Read the model definition and answer for the solid it produces. Units are mm, in the model's axes. Give positions to 0.01 mm unless a question says otherwise; leave off trailing zeros. Order: outer loops, then holes, each group sorted by start corner. A loop starts at its lowest first (then second) coordinate and runs counter-clockwise, first axis right, second up.
```python
from build123d import *

# Parameters (mm, degrees)
SKETCH1_W           = 203.2
SKETCH1_H           = 133.35
BOSS_EXTRUDE1_DEPTH = 3.175
SKETCH3_W           = 35.687
SKETCH3_H           = 3.175
BOSS_EXTRUDE2_DEPTH = 3.175
SKETCH4_W           = 3.175
SKETCH4_H           = 18.542
BOSS_EXTRUDE3_DEPTH = 3.175
SKETCH5_W           = 63.5
SKETCH5_H           = 139.7
SKETCH5_R           = 3.429
BOSS_EXTRUDE4_DEPTH = 3.175
BOSS_EXTRUDE5_DEPTH = 3.175
SKETCH7_W           = 3.683
SKETCH7_H           = 19.558
CUT_EXTRUDE1_DEPTH  = 183.223979624
SKETCH8_W           = 71.12
SKETCH8_H           = 45.72
CUT_EXTRUDE4_DEPTH  = 183.223979624


with BuildPart() as part:
    # Sketch1 → Boss-Extrude1 (new body)
    with BuildSketch(Plane(origin=(0, 0, 0), x_dir=(1, 0, 0), z_dir=(0, 1, 0))):
        Rectangle(SKETCH1_W, SKETCH1_H)
    extrude(amount=BOSS_EXTRUDE1_DEPTH)

    # Sketch3 → Boss-Extrude2 (add)
    with BuildSketch(Plane(origin=(0, 3.175, 0), x_dir=(1, 0, 0), z_dir=(0, 1, 0))):
        with Locations((-61.2775, 68.2625)):
            Rectangle(SKETCH3_W, SKETCH3_H)
        with Locations((0.3175, 68.2625)):
            Rectangle(SKETCH3_W, SKETCH3_H)
        with Locations((61.9125, 68.2625)):
            Rectangle(SKETCH3_W, SKETCH3_H)
        with Locations((61.9125, -68.2625)):
            Rectangle(SKETCH3_W, SKETCH3_H)
        with Locations((0.3175, -68.2625)):
            Rectangle(SKETCH3_W, SKETCH3_H)
        with Locations((-61.2775, -68.2625)):
            Rectangle(SKETCH3_W, SKETCH3_H)
    extrude(amount=-BOSS_EXTRUDE2_DEPTH)

    # Sketch4 → Boss-Extrude3 (add)
    with BuildSketch(Plane(origin=(0, 3.175, 0), x_dir=(1, 0, 0), z_dir=(0, 1, 0))):
        with Locations((-103.1875, 38.1)):
            Rectangle(SKETCH4_W, SKETCH4_H)
        with Locations((-103.1875, 0)):
            Rectangle(SKETCH4_W, SKETCH4_H)
        with Locations((-103.1875, -38.1)):
            Rectangle(SKETCH4_W, SKETCH4_H)
        with Locations((103.1875, -38.1)):
            Rectangle(SKETCH4_W, SKETCH4_H)
        with Locations((103.1875, 0)):
            Rectangle(SKETCH4_W, SKETCH4_H)
        with Locations((103.1875, 38.1)):
            Rectangle(SKETCH4_W, SKETCH4_H)
    extrude(amount=-BOSS_EXTRUDE3_DEPTH)

    # Sketch5 → Boss-Extrude4 (add)
    with BuildSketch(Plane(origin=(0, 3.175, 0), x_dir=(1, 0, 0), z_dir=(0, 1, 0))):
        with Locations((-136.525, 0)):
            Rectangle(SKETCH5_W, SKETCH5_H)
        with Locations(Location((-117.475, 57.15, 0), (0, 0, 270))):
            Circle(SKETCH5_R, mode=Mode.SUBTRACT)
        with Locations(Location((-130.175, 57.15, 0), (0, 0, 270))):
            Circle(SKETCH5_R, mode=Mode.SUBTRACT)
        with Locations(Location((-142.875, 57.15, 0), (0, 0, 270))):
            Circle(SKETCH5_R, mode=Mode.SUBTRACT)
        with Locations(Location((-155.575, 57.15, 0), (0, 0, 270))):
            Circle(SKETCH5_R, mode=Mode.SUBTRACT)
        with Locations(Location((-130.175, 44.45, 0), (0, 0, 270))):
            Circle(SKETCH5_R, mode=Mode.SUBTRACT)
        with Locations(Location((-142.875, 44.45, 0), (0, 0, 270))):
            Circle(SKETCH5_R, mode=Mode.SUBTRACT)
        with Locations(Location((-155.575, 44.45, 0), (0, 0, 270))):
            Circle(SKETCH5_R, mode=Mode.SUBTRACT)
        with Locations(Location((-130.175, 31.75, 0), (0, 0, 270))):
            Circle(SKETCH5_R, mode=Mode.SUBTRACT)
        with Locations(Location((-142.875, 31.75, 0), (0, 0, 270))):
            Circle(SKETCH5_R, mode=Mode.SUBTRACT)
        with Locations(Location((-155.575, 31.75, 0), (0, 0, 270))):
            Circle(SKETCH5_R, mode=Mode.SUBTRACT)
        with Locations(Location((-130.175, 19.05, 0), (0, 0, 270))):
            Circle(SKETCH5_R, mode=Mode.SUBTRACT)
        with Locations(Location((-142.875, 19.05, 0), (0, 0, 270))):
            Circle(SKETCH5_R, mode=Mode.SUBTRACT)
        with Locations(Location((-155.575, 19.05, 0), (0, 0, 270))):
            Circle(SKETCH5_R, mode=Mode.SUBTRACT)
        with Locations(Location((-130.175, 6.35, 0), (0, 0, 270))):
            Circle(SKETCH5_R, mode=Mode.SUBTRACT)
        with Locations(Location((-142.875, 6.35, 0), (0, 0, 270))):
            Circle(SKETCH5_R, mode=Mode.SUBTRACT)
        with Locations(Location((-155.575, 6.35, 0), (0, 0, 270))):
            Circle(SKETCH5_R, mode=Mode.SUBTRACT)
        with Locations(Location((-130.175, -6.35, 0), (0, 0, 270))):
            Circle(SKETCH5_R, mode=Mode.SUBTRACT)
        with Locations(Location((-142.875, -6.35, 0), (0, 0, 270))):
            Circle(SKETCH5_R, mode=Mode.SUBTRACT)
        with Locations(Location((-155.575, -6.35, 0), (0, 0, 270))):
            Circle(SKETCH5_R, mode=Mode.SUBTRACT)
        with Locations(Location((-130.175, -19.05, 0), (0, 0, 270))):
            Circle(SKETCH5_R, mode=Mode.SUBTRACT)
        with Locations(Location((-142.875, -19.05, 0), (0, 0, 270))):
            Circle(SKETCH5_R, mode=Mode.SUBTRACT)
        with Locations(Location((-155.575, -19.05, 0), (0, 0, 270))):
            Circle(SKETCH5_R, mode=Mode.SUBTRACT)
        with Locations(Location((-130.175, -31.75, 0), (0, 0, 270))):
            Circle(SKETCH5_R, mode=Mode.SUBTRACT)
        with Locations(Location((-142.875, -31.75, 0), (0, 0, 270))):
            Circle(SKETCH5_R, mode=Mode.SUBTRACT)
        with Locations(Location((-155.575, -31.75, 0), (0, 0, 270))):
            Circle(SKETCH5_R, mode=Mode.SUBTRACT)
        with Locations(Location((-130.175, -44.45, 0), (0, 0, 270))):
            Circle(SKETCH5_R, mode=Mode.SUBTRACT)
        with Locations(Location((-142.875, -44.45, 0), (0, 0, 270))):
            Circle(SKETCH5_R, mode=Mode.SUBTRACT)
        with Locations(Location((-155.575, -44.45, 0), (0, 0, 270))):
            Circle(SKETCH5_R, mode=Mode.SUBTRACT)
        with Locations(Location((-130.175, -57.15, 0), (0, 0, 270))):
            Circle(SKETCH5_R, mode=Mode.SUBTRACT)
        with Locations(Location((-142.875, -57.15, 0), (0, 0, 270))):
            Circle(SKETCH5_R, mode=Mode.SUBTRACT)
        with Locations(Location((-155.575, -57.15, 0), (0, 0, 270))):
            Circle(SKETCH5_R, mode=Mode.SUBTRACT)
        with Locations(Location((-117.475, 44.45, 0), (0, 0, 270))):
            Circle(SKETCH5_R, mode=Mode.SUBTRACT)
        with Locations(Location((-117.475, 31.75, 0), (0, 0, 270))):
            Circle(SKETCH5_R, mode=Mode.SUBTRACT)
        with Locations(Location((-117.475, 19.05, 0), (0, 0, 270))):
            Circle(SKETCH5_R, mode=Mode.SUBTRACT)
        with Locations(Location((-117.475, 6.35, 0), (0, 0, 270))):
            Circle(SKETCH5_R, mode=Mode.SUBTRACT)
        with Locations(Location((-117.475, -6.35, 0), (0, 0, 270))):
            Circle(SKETCH5_R, mode=Mode.SUBTRACT)
        with Locations(Location((-117.475, -19.05, 0), (0, 0, 270))):
            Circle(SKETCH5_R, mode=Mode.SUBTRACT)
        with Locations(Location((-117.475, -31.75, 0), (0, 0, 270))):
            Circle(SKETCH5_R, mode=Mode.SUBTRACT)
        with Locations(Location((-117.475, -44.45, 0), (0, 0, 270))):
            Circle(SKETCH5_R, mode=Mode.SUBTRACT)
        with Locations(Location((-117.475, -57.15, 0), (0, 0, 270))):
            Circle(SKETCH5_R, mode=Mode.SUBTRACT)
    extrude(amount=-BOSS_EXTRUDE4_DEPTH)

    # Sketch6 → Boss-Extrude5 (add)
    with BuildSketch(Plane(origin=(0, 3.175, 0), x_dir=(1, 0, 0), z_dir=(0, 1, 0))):
        Polygon((-79.121, 66.675), (-79.121, 69.85), (-104.775, 69.85), (-104.775, 58.6105), (-104.775, 47.371), (-101.6, 47.371), (-101.6, 66.675), align=None)
        Polygon((-104.775, -47.371), (-104.775, -58.6105), (-104.775, -69.85), (-79.121, -69.85), (-79.121, -66.675), (-101.6, -66.675), (-101.6, -47.371), align=None)
        Polygon((79.121, -66.675), (79.121, -69.85), (104.775, -69.85), (104.775, -58.6105), (104.775, -47.371), (101.6, -47.371), (101.6, -66.675), align=None)
        Polygon((104.775, 47.371), (104.775, 58.6105), (104.775, 69.85), (79.121, 69.85), (79.121, 66.675), (101.6, 66.675), (101.6, 47.371), align=None)
    extrude(amount=-BOSS_EXTRUDE5_DEPTH)

    # Sketch7 → Cut-Extrude1 (cut, through all)
    with BuildSketch(Plane(origin=(0, 3.175, 0), x_dir=(1, 0, 0), z_dir=(0, 1, 0))):
        with Locations((-103.1875, 19.05)):
            Rectangle(SKETCH7_W, SKETCH7_H)
        with Locations((-103.1875, -19.05)):
            Rectangle(SKETCH7_W, SKETCH7_H)
    extrude(amount=-CUT_EXTRUDE1_DEPTH, mode=Mode.SUBTRACT)

    # Sketch8 → Cut-Extrude4 (cut, through all)
    with BuildSketch(Plane(origin=(0, 0, 0), x_dir=(1, 0, 0), z_dir=(0, 1, 0))):
        with Locations((50.8, 0)):
            Rectangle(SKETCH8_W, SKETCH8_H)
    extrude(amount=CUT_EXTRUDE4_DEPTH, mode=Mode.SUBTRACT)


solid = part.part
```
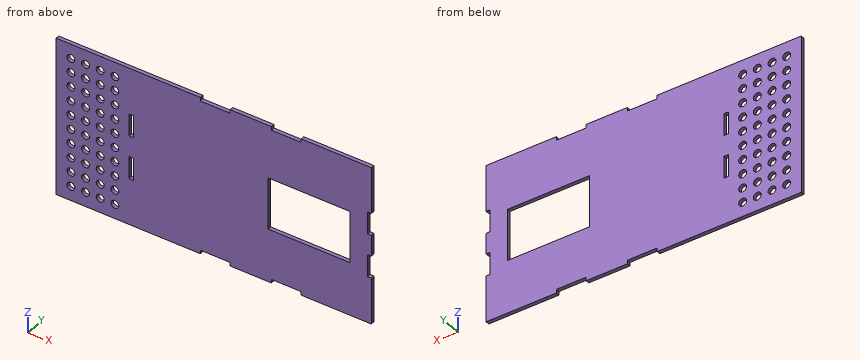
1) The part is cut by section B-B on z = 19.05. Determine the outline of the cut face in (x, y) (3 decimals).
Final values:
outline: (-168.275, 0) - (-159.004, 0) - (-159.004, 3.175) - (-168.275, 3.175) - close; (-152.146, 0) - (-146.304, 0) - (-146.304, 3.175) - (-152.146, 3.175) - close; (-139.446, 0) - (-133.604, 0) - (-133.604, 3.175) - (-139.446, 3.175) - close; (-126.746, 0) - (-120.904, 0) - (-120.904, 3.175) - (-126.746, 3.175) - close; (-114.046, 0) - (-105.029, 0) - (-105.029, 3.175) - (-114.046, 3.175) - close; (-101.346, 0) - (15.24, 0) - (15.24, 3.175) - (-101.346, 3.175) - close; (86.36, 0) - (101.6, 0) - (101.6, 3.175) - (86.36, 3.175) - close
2) The part is cut by section A-A on x = 21.5. Determine the outline of the cut face in (y, z) (3 decimals).
Final values:
outline: (0, -66.675) - (3.175, -66.675) - (3.175, -22.86) - (0, -22.86) - close; (0, 22.86) - (3.175, 22.86) - (3.175, 66.675) - (0, 66.675) - close
3) Consider L1, parallel to X at y = 0.85, z = -6.35 (3 decimals); L2, parallel to X at y = 1.8, z = 44.45 (3 decimals); L3, parallel to X at y = 0.15, z = 12 (3 decimals). Determine where each line is inside the solid, lowest interval first.
Final values:
L1: x = -168.275 to -159.004, -152.146 to -146.304, -139.446 to -133.604, -126.746 to -120.904, -114.046 to 15.24, 86.36 to 104.775
L2: x = -168.275 to -159.004, -152.146 to -146.304, -139.446 to -133.604, -126.746 to -120.904, -114.046 to 104.775
L3: x = -168.275 to -105.029, -101.346 to 15.24, 86.36 to 101.6
4) The part is cut by section D-D on x = 65. Determine the outline of the cut face in (y, z) (3 decimals), and give its area (3 significant figures).
Final values:
outline: (0, -69.85) - (3.175, -69.85) - (3.175, -22.86) - (0, -22.86) - close; (0, 22.86) - (3.175, 22.86) - (3.175, 69.85) - (0, 69.85) - close
area: 298 mm2
5) Given pin 1 (9 mm diameter, centred on x = -142.875, z = -19.05, fed in from +Y) (3 decimals), flat-ended and moving along its own axis, determine where the tip first touches the part or whether it passes through.
Final values:
pin 1: stops at y = 3.175
6) The part is cut by section C-C on z = -31.75. Determine the outline of the cut face in (x, y) (3 decimals).
Final values:
outline: (-168.275, 0) - (-159.004, 0) - (-159.004, 3.175) - (-168.275, 3.175) - close; (-152.146, 0) - (-146.304, 0) - (-146.304, 3.175) - (-152.146, 3.175) - close; (-139.446, 0) - (-133.604, 0) - (-133.604, 3.175) - (-139.446, 3.175) - close; (-126.746, 0) - (-120.904, 0) - (-120.904, 3.175) - (-126.746, 3.175) - close; (-114.046, 0) - (104.775, 0) - (104.775, 3.175) - (-114.046, 3.175) - close
